```python
from build123d import *

# Parameters (mm, degrees)
F0_R     = 18.25
F1_DEPTH = 28


# Not quite as in the source:
# - a feature names something its author has since deleted; it is built from what else it names


with BuildPart() as f1:
    # F0 (on Top) → F1 (new body)
    with BuildSketch(Plane.XY):
        with BuildLine():
            Line((23.5539685776, 114.0594776705), (23.1539685776, 114.0594776705))
            ThreePointArc((23.1539685776, 114.0594776705), (-6.7566482666, 101.6700945147), (-19.1460314224, 71.7594776705))
            Line((-19.1460314224, 71.7594776705), (-19.1460314224, 40.5602956202))
            ThreePointArc((-19.1460314224, 40.5602956202), (-18.8100234812, 35.3865412816), (-17.8076447246, 30.2997080702))
            ThreePointArc((-17.8076447246, 30.2997080702), (-10.7929031817, -17.2712382489), (-14.6173474127, -65.2042660996))
            ThreePointArc((-14.6173474127, -65.2042660996), (-15.16027858, -71.7938854137), (-14.2465279536, -78.3423903385))
            ThreePointArc((-14.2465279536, -78.3423903385), (24.3685631197, -108.3214348669), (62.983654193, -78.3423903385))
            ThreePointArc((62.983654193, -78.3423903385), (63.6357145351, -72.9718093248), (62.983654193, -67.6012283111))
            ThreePointArc((62.983654193, -67.6012283111), (62.8457925436, -65.8846278256), (62.6096584736, -64.1787662362))
            ThreePointArc((62.6096584736, -64.1787662362), (59.2183076196, -16.4494096847), (64.932743293, 31.0578314726))
            ThreePointArc((64.932743293, 31.0578314726), (65.6229953988, 35.3006378942), (65.8539685776, 39.593015521))
            Line((65.8539685776, 39.593015521), (65.8539685776, 71.7594776705))
            ThreePointArc((65.8539685776, 71.7594776705), (53.4645854218, 101.6700945147), (23.5539685776, 114.0594776705))
        make_face()
        with Locations((25.6633214675, -68.4624532511)):
            Circle(F0_R, mode=Mode.SUBTRACT)
    extrude(amount=F1_DEPTH)


solid = f1.part
```
Source: CAD feature listing. Evaluate the final solid. Frame: model axes, mm. Round coordinates to 2 decimals unless told otherwise and drop trailing zeros. Loops run counter-clockwise (first coordinate to the right, second up) from the corner with the lowest first, then second, coordinate; pieces in that order, holes last. Notation, with made-up numbers: M 75,-29 L 115,-29 A34 cw 115,5 Z; hole C -15,46.25 d4. An arc over 180 degrees is marked long. Use a Markdown table: item, result. Add a question column.
1. Mould query, pull axis Y, two halves, no side actions, for faces 1 (the flat face through (65.854, 55, 14)), 2 (the cylindrical face through (-6.426, 101.997, 13.804)), 3 (the cylindrical face through (-15.163, -71.701, 13.804)). Classes: pulls with the +Y half, pulls with the -Y half, needs draft (parallel to the pull), parting line crosses it, or undercut.
2. Line query: line 1 (X direction, y = -53, z = 11.5); line 2 (X direction, y = -21, z = 7.25); line 3 (Y direction, x = 31.5, z = 26.5). Output: solid intervals per line, ascending.
3. Section query C-C on y = -58.5. Return the cut outline in (x, z).
4. Contact query for flat-ended pins moving along their axis: P1, Ø2, axis at y = -85.5, z = 4, coming from the -X side; P2, Ø1.5, axis at x = 25, z = 5, coming from the +Y side; P3, Ø10, axis at x = 56.5, z = 7.5, coming from the -Y side. Output: stop coordinate, or through.
5. Section query D-D on x = -4. Return the cut outline in (y, z), then the cut area to 3 significant figures.
6. Section query B-B on z = 24.5. Return the cut outline in (x, y), then the cut area to 3 significant figures.
7. Section query A-A on x = 14.5. Return the cut outline in (y, z), then the cut area to 3 significant figures.
Reported:
| question | item | result |
|---|---|---|
| 1 | face 1 | needs draft |
| 1 | face 2 | pulls with the +Y half |
| 1 | face 3 | undercut |
| 2 | line 1 | x = -12.6 to 15.97, 35.36 to 60.99 |
| 2 | line 2 | x = -10.7 to 59.15 |
| 2 | line 3 | y = -107.68 to -85.75, -51.17 to 113.31 |
| 3 | outline | M -13.42,0 L 10.37,0 L 10.37,28 L -13.42,28 Z; M 40.95,0 L 61.72,0 L 61.72,28 L 40.95,28 Z |
| 4 | P1 | stops at x = -12.12 |
| 4 | P2 | stops at y = 114.05 |
| 4 | P3 | stops at y = -97.66 |
| 5 | outline | M -96.46,0 L 104.19,0 L 104.19,28 L -96.46,28 Z |
| 5 | area | 5,620 mm² |
| 6 | outline | M -19.15,40.56 A40 ccw -17.81,30.3 A213.2 cw -14.62,-65.2 A30 ccw -14.25,-78.34 A39.86 ccw 62.98,-78.34 A22.44 ccw 62.98,-67.6 A30 ccw 62.61,-64.18 A251.37 cw 64.93,31.06 A40 ccw 65.85,39.59 L 65.85,71.76 A42.3 ccw 23.55,114.06 L 23.15,114.06 A42.3 ccw -19.15,71.76 Z; hole C 25.66,-68.46 d36.5 |
| 6 | area | 15,000 mm² |
| 7 | outline | M -107.08,0 L -82.9,0 L -82.9,28 L -107.08,28 Z; M -54.02,0 L 113.16,0 L 113.16,28 L -54.02,28 Z |
| 7 | area | 5,360 mm² |
